Read the model definition and answer for the solid it produces. Units are mm, in the model's axes. A direction names the side the tool comes from. Round coordinates to 2 decimals unless told otherwise and drop trailing zeros. Order: outer loops, then holes, each group sorted by start corner. A loop starts at its lowest first (then second) coordinate and runs counter-clockwise, first axis right, second up. Notation, with made-up numbers: (84.25, -13) - (124.25, -13) arc R24 cw to (124.25, 13) - close; hole circle Ø4 at (-29.5, 67.25). An arc over 180 degrees is marked (long way). One line per question, with ' | ' between items. Start each with the question number.
1) The part is cut by section A-A, the plane z = 503. Give the vertices of the cut face in (x, y), plus the area to 3 significant figures.
2) The part is cut by section C-C, the plane y = -211. Give the vertices of the cut face in (x, z).
3) Flat-ended cylindrical pins translate along their axes: pin 1 (10 mm diameter, centred on x = 214.5, z = 668.5, fed in from -Y); pin 2 (6 mm diameter, centred on x = 267.5, y = -705.5, fed in from +Z). Find the tip coordinate at first contact, or state that the pin passes through.
4) Straight lines are drawn through the part: line 1 (X direction, y = -564.5, z = 629); line 2 (Y direction, x = 739.5, z = 720); line 3 (Z direction, x = 864.5, y = -733). For each, find the intervals that lie inside material, in ascending order. Write a range as from..to.
5) The mould has two halves that part along X. Classify faces 4 (the flat face through (751, -152.4, 594)), 5 (the flat face through (751, -401, 0)), 6 (the flat face through (753, -478, 381)), 7 (the flat face through (0, -412, 310)): pulls with the +X half, pulls with the -X half, needs draft (parallel to the pull), parting line crosses it, or undercut.
6) The part is cut by section D-D, the plane x = 109.5. Give the vertices of the cut face in (y, z).
7) For faces 1 (the flat face through (751, -812.8, 242)), 2 (the flat face through (152.4, -487, 506)), 3 (the flat face through (75, -478, 635)), determine the directions among +Z, -Z, +X, -X, +Y, -Y from which every point of the face is accessible in a straight line to the end or side of a thin tool.
8) The part is cut by section B-B, the plane x = 820. Give the vertices of the cut face in (y, z), plus the area to 3 significant figures.
from build123d import *

# Parameters (mm, degrees)
F0_W     = 1524
F0_H     = 812.8
F1_DEPTH = 381
F3_DEPTH = 254
F4_W     = 1524
F4_H     = 152.4
F5_DEPTH = 177.8


with BuildPart() as f1:
    # F0 (on Top) → F1 (new body)
    with BuildSketch(Plane.XY):
        with Locations((762, -406.4)):
            Rectangle(F0_W, F0_H)
    extrude(amount=F1_DEPTH)

    # F2 (on face) → F3 (join)
    with BuildSketch(Plane.XY.offset(381)):
        Polygon((0, 0), (0, -812.8), (152.4, -812.8), (152.4, -152.4), (1371.6, -152.4), (1371.6, -812.8), (1524, -812.8), (1524, 0), align=None)
    extrude(amount=F3_DEPTH)

    # F4 (on face) → F5 (join)
    with BuildSketch(Plane.XY.offset(635)):
        with Locations((762, -76.2)):
            Rectangle(F4_W, F4_H)
    extrude(amount=F5_DEPTH)


solid = f1.part
Values:
1) outline: (0, -812.8) - (152.4, -812.8) - (152.4, -152.4) - (1371.6, -152.4) - (1371.6, -812.8) - (1524, -812.8) - (1524, 0) - (0, 0) - close | area: 434,000 mm^2
2) outline: (0, 0) - (1524, 0) - (1524, 635) - (1371.6, 635) - (1371.6, 381) - (152.4, 381) - (152.4, 635) - (0, 635) - close
3) pin 1: stops at y = -152.4 | pin 2: stops at z = 381
4) line 1: x = 0..152.4, 1371.6..1524 | line 2: y = -152.4..0 | line 3: z = 0..381
5) face 4: undercut | face 5: needs draft | face 6: undercut | face 7: pulls with the -X half
6) outline: (-812.8, 0) - (0, 0) - (0, 812.8) - (-152.4, 812.8) - (-152.4, 635) - (-812.8, 635) - close
7) face 1: +Z, -Z, +X, -X, -Y | face 2: +Z, -Y | face 3: +Z, +X, -X, -Y
8) outline: (-812.8, 0) - (0, 0) - (0, 812.8) - (-152.4, 812.8) - (-152.4, 381) - (-812.8, 381) - close | area: 375,000 mm^2
